Autodesk Fusion 360 part; units mm, degrees
sketch "Sketch1" plane through (0, 0, 0) normal (0, 0, 1) x (1, 0, 0)
  circle A0 centre (0, 65) radius 10
  circle A1 centre (-47, -26) radius 7
  arc A2 (-27.0298, 18.9312) -> (-15.8903, 63.1292) centre (-79.4513, 55.6462) ccw
  circle A3 centre (-0.1967, -50) radius 5
  arc A4 (-48.9633, -16.1946) -> (-32.9314, 2.127) centre (-52.8898, 3.4162) ccw
  arc A5 (-9.9929, -47.9913) -> (-18.421, -27.38) centre (-29.5853, -43.974) ccw
  arc A6 (-21.5665, -24.9777) -> (-37.5509, -29.2733) centre (-28.1018, -32.5467) ccw
  arc A7 (-19.1, -5.9321) -> (-19.1, 5.9321) centre (-20, 0) ccw
  arc A8 (-19.1, -5.9321) -> (-19.1, 5.9321) centre (-20, 0) ccw
  arc A9 (-19.1, -5.9321) -> (-19.1, 5.9321) centre (-20, 0) ccw
  arc A10 (-19.1, -5.9321) -> (-19.1, 5.9321) centre (-20, 0) ccw
  arc A11 (-4.4126, -19.5071) -> (-14.6874, -13.575) centre (-10, -17.3205) ccw
  arc A12 (14.6874, -13.575) -> (4.4126, -19.5071) centre (10, -17.3205) ccw
  arc A13 (-19.1, -5.9321) -> (-19.1, 5.9321) centre (-20, 0) ccw
  arc A14 (-19.1, -5.9321) -> (-14.6874, -13.575) centre (0, 0) ccw
  arc A15 (-14.6874, 13.575) -> (-4.4126, 19.5071) centre (-10, 17.3205) ccw
  arc A16 (-14.6874, 13.575) -> (-19.1, 5.9321) centre (0, 0) ccw
  arc A17 (4.4126, 19.5071) -> (14.6874, 13.575) centre (10, 17.3205) ccw
  arc A18 (4.4126, 19.5071) -> (-4.4126, 19.5071) centre (0, 0) ccw
  arc A19 (19.1, 5.9321) -> (19.1, -5.9321) centre (20, 0) ccw
  arc A20 (19.1, 5.9321) -> (14.6874, 13.575) centre (0, 0) ccw
  arc A21 (-4.4126, -19.5071) -> (4.4126, -19.5071) centre (0, 0) ccw
  arc A22 (14.6874, -13.575) -> (19.1, -5.9321) centre (0, 0) ccw
  arc A23 (-19.1, -5.9321) -> (-19.1, 5.9321) centre (-20, 0) ccw
  circle A24 centre (0, 65) radius 10
  arc A25 (15.8903, 63.1292) -> (27.0298, 18.9312) centre (79.4513, 55.6462) ccw
  arc A26 (32.9314, 2.127) -> (48.9633, -16.1946) centre (52.8898, 3.4162) ccw
  circle A27 centre (47, -26) radius 7
  arc A28 (37.5509, -29.2733) -> (21.5665, -24.9777) centre (28.1018, -32.5467) ccw
  arc A29 (18.421, -27.38) -> (9.9929, -47.9913) centre (29.5853, -43.974) ccw
  arc A30 (14.6874, -13.575) -> (19.1, -5.9321) centre (0, 0) ccw
  arc A31 (19.1, 5.9321) -> (19.1, -5.9321) centre (20, 0) ccw
  arc A32 (19.1, 5.9321) -> (14.6874, 13.575) centre (0, 0) ccw
  arc A33 (4.4126, 19.5071) -> (14.6874, 13.575) centre (10, 17.3205) ccw
  arc A34 (4.4126, 19.5071) -> (-4.4126, 19.5071) centre (0, 0) ccw
  arc A35 (-4.4126, -19.5071) -> (4.4126, -19.5071) centre (0, 0) ccw
  arc A36 (14.6874, -13.575) -> (4.4126, -19.5071) centre (10, -17.3205) ccw
  circle A37 centre (0.1967, -50) radius 5
  arc A38 (-4.4126, -19.5071) -> (-14.6874, -13.575) centre (-10, -17.3205) ccw
  arc A39 (-19.1, -5.9321) -> (-14.6874, -13.575) centre (0, 0) ccw
  arc A40 (-19.1, -5.9321) -> (-19.1, 5.9321) centre (-20, 0) ccw
  arc A41 (-14.6874, 13.575) -> (-4.4126, 19.5071) centre (-10, 17.3205) ccw
  arc A42 (-14.6874, 13.575) -> (-19.1, 5.9321) centre (0, 0) ccw
  arc A43 (-27.0298, 18.9312) -> (-32.9314, 2.127) centre (0, 0) ccw
  arc A44 (-27.0298, 18.9312) -> (-32.9314, 2.127) centre (0, 0) ccw
  arc A45 (-21.5665, -24.9777) -> (-18.421, -27.38) centre (0, 0) ccw
  arc A46 (-21.5665, -24.9777) -> (-18.421, -27.38) centre (0, 0) ccw
  arc A47 (18.421, -27.38) -> (21.5665, -24.9777) centre (0, 0) ccw
  arc A48 (32.9314, 2.127) -> (27.0298, 18.9312) centre (0, 0) ccw
  arc A49 (18.421, -27.38) -> (21.5665, -24.9777) centre (0, 0) ccw
  arc A50 (32.9314, 2.127) -> (27.0298, 18.9312) centre (0, 0) ccw
  arc A51 (-9.9929, -47.9913) -> (0, -59.9981) centre (-0.1967, -50) ccw
  arc A52 (0, -59.9981) -> (9.9929, -47.9913) centre (0.1967, -50) ccw
  arc A53 (-48.9633, -16.1946) -> (-37.5509, -29.2733) centre (-47, -26) ccw
  arc A54 (37.5509, -29.2733) -> (48.9633, -16.1946) centre (47, -26) ccw
  arc A55 (15.8903, 63.1292) -> (-15.8903, 63.1292) centre (0, 65) ccw
  arc A56 (15.8903, 63.1292) -> (-15.8903, 63.1292) centre (0, 65) ccw
  dimension "d1" = 20
  dimension "d2" = 65
  dimension "d3" = 32
  dimension "d4" = 40
  dimension "d5" = 66
  dimension "d6" = 128
  dimension "d7" = 14
  dimension "d8" = 47
  dimension "d9" = 26
  dimension "d10" = 20
  dimension "d11" = 40
  dimension "d12" = 10
  dimension "d13" = 50
  dimension "d14" = 20
  dimension "d15" = 40
  dimension "d16" = 20
  dimension "d17" = 12
  dimension "d21" = 360
sketch "Sketch2" plane through (0, 0, 0) normal (0, 0, 1) x (1, 0, 0)
sketch "Sketch3" plane through (0, 0, 0) normal (0, 0, 1) x (1, 0, 0)
extrude "Extrude1" add sketch "Sketch1" along normal blind 50
Verification items for the finished model (mm, model axes). A direction names the side the tool comes from. Coordinates: 2 decimals unless noted, no trailing zeros. Order: outer loops, then holes, each group sorted by start corner. A loop starts at its lowest first (then second) coordinate and runs counter-clockwise, first axis right, second up. Notation, with made-up numbers: M 54.5,17.5 L 76.5,17.5 A15 cw 76.5,27.5 Z; hole C 46.5,31 d9. An arc over 180 degrees is marked long. One line per item, written item: value. Start each with the question number.
Item 1: Sectioned sample at D-D (y = 28.5). Enter the section's corners in (x, z).
Item 2: Sectioned sample at A-A (y = 65). Enter the section's corners in (x, z).
Item 3: Sectioned sample at C-C (z = 25.5). Count the separate pieces of the cut face and the enclosed holes in it, then the cut area to 3 significant figures.
Item 4: Mould release check, pull along X, two halves, no side actions. Record for faces 4 (the cylindrical face through (-37.72, -9.62, 24.65)), 5 (the cylindrical face through (17.35, -9.95, 24.65)), 6 (the flat face through (-4.5, 16.1, 0)): released by +X, released by -X, zero draft, split by the parting line, or undercut.
Item 5: Scan lines: probe 1 along Y at (x, z) = (0, 11.5); probe 2 along X at (y, z) = (65.5, 3); probe 3 along Y at (x, z) = (2, 2). Record each from-to range of solid material in increasing order.
Item 6: Access from +Z, -Z, +X, -X, +Y, -Y to the whole of each face (thin tool, end or side, straight path). Record for faces 1 (the cylindrical face through (5.195, -49.887, 24.65)), 2 (the cylindrical face through (17.473, 39.689, 24.65)), 3 (the cylindrical face through (20.05, -26.21, 24.65)).
Item 7: Sectioned sample at B-B (y = -50). Enter the section's corners in (x, z).
Item 8: Gauge pin test, flat ends, axial feed: pin 1 (3 mm diameter, centred on x = 28.5, z = 24, fed in from -Y); pin 2 (4 mm diameter, centred on y = -41.5, z = 34, fed in from -X); pin 3 (5 mm diameter, centred on x = 15.5, z = 22.5, fed in from +Y). Record the tip position at first contact, or that the pin passes through.
Conclusion:
1. outline: M -21.49,0 L 21.49,0 L 21.49,50 L -21.49,50 Z
2. outline: M -16,0 L -10,0 L -10,50 L -16,50 Z; M 10,0 L 16,0 L 16,50 L 10,50 Z
3. separate pieces: 1
3. enclosed holes: 5
3. area: 4,920 mm^2
4. face 4: released by -X
4. face 5: undercut
4. face 6: zero draft
5. probe 1: y = -60 to -55, -45 to -20, 20 to 55, 75 to 81
5. probe 2: x = -15.99 to -9.99, 9.99 to 15.99
5. probe 3: y = -59.84 to -54.66, -45.34 to -19.9, 19.9 to 55.2, 74.8 to 80.87
6. face 1: +Z, -Z
6. face 2: +Z, -Z, +X
6. face 3: +Z, -Z, -Y
7. outline: M -10.2,0 L -5.2,0 L -5.2,50 L -10.2,50 Z; M 5.2,0 L 10.2,0 L 10.2,50 L 5.2,50 Z
8. pin 1: stops at y = -22.73
8. pin 2: stops at x = -10.09
8. pin 3: stops at y = 74.33
